Source: three-view drawing plus pictorial views. Frame: mm from the lowest corner of the part. A direction names the side the tool comes from. Round coordinates to 2 decimals unless told otherwise and drop trailing zeros. Order: outer loops, then holes, each group sorted by start corner. A loop starts at its lowest first (then second) coordinate and runs counter-clockwise, first axis right, second up. Notation, with made-up numbers: M 38,79 L 42,79 A18 cw 42,90 Z; hole C 48,10 d6. An arc over 180 degrees is marked long. Return JSON: item names as keys, results as strings. Group by question number.
Q1. Mould query, pull axis Y, two halves, no side actions, for the marked faces 1, 2 and 3. Classes: released by +Y, released by -Y, zero draft, split by the parting line, or undercut.
Q2. Ray query, probe 1 along Y at (x, z) = (12, 4.25); probe 2 along X at (y, z) = (11, 1.5); probe 3 along Y at (x, z) = (70, 0.75). Return the intervals inside material, ascending.
Q3. Access query for the marked faces 4 and 5. Directions: +Z, -Z, +X, -X, +Y, -Y. A direction counts if a zero-diameter tool reaches every point of the face in a straight line with its end or side. Return the directions, or none.
Q4. Cut plane D-D on x = 23.5. Output: boundary loops of the cut face in (y, z), and give its area (3 significant figures).
Q5. Contact query for flat-ended pins moving along their axis: pin 1 (1 mm diameter, centred on x = 31, y = 17.5, fed in from +Z); pin 2 (3.5 mm diameter, centred on x = 45, y = 12.5, fed in from +Z). Output: stop coordinate, or through.
Q6. Cut plane B-B on z = 20. Output: boundary loops of the cut face in (x, y).
Q7. Cut plane C-C on x = 35. Output: boundary loops of the cut face in (y, z).
Q8. Cut plane A-A on y = 12.5. Output: boundary loops of the cut face in (x, z), and give its area (3 significant figures).
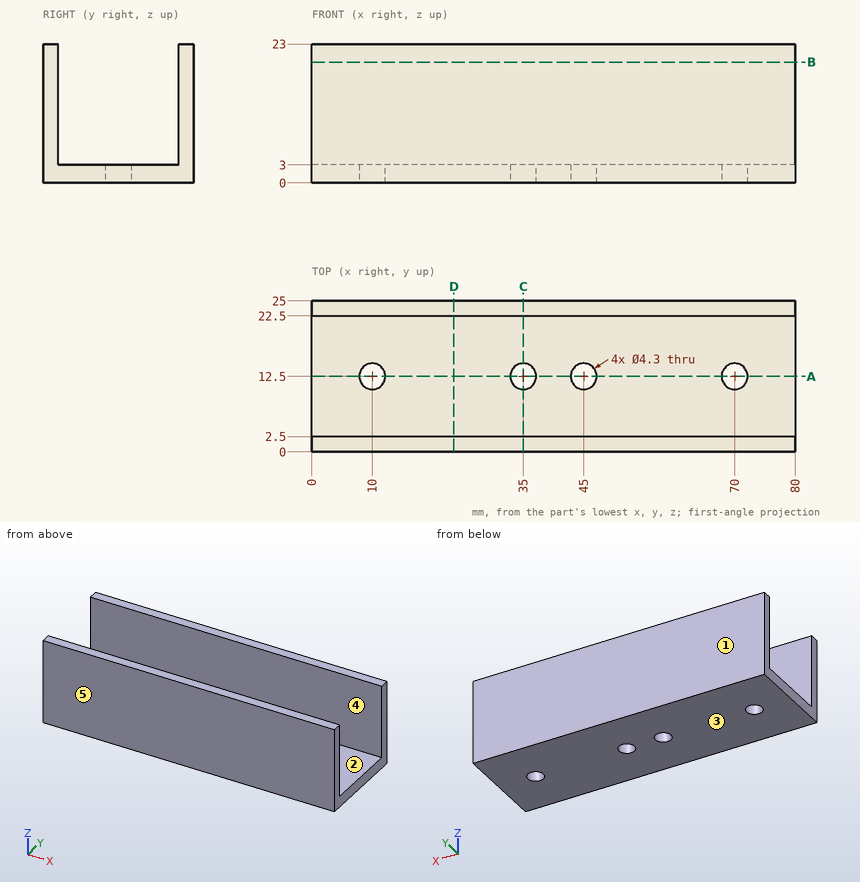
Result sheet:
{
 "1": {"face 1": "released by +Y", "face 2": "undercut", "face 3": "zero draft"},
 "2": {"probe 1": "y = 0 to 2.5, 22.5 to 25", "probe 2": "x = 0 to 8.46, 11.54 to 33.46, 36.54 to 43.46, 46.54 to 68.46, 71.54 to 80", "probe 3": "y = 0 to 10.35, 14.65 to 25"},
 "3": {"face 4": "+Z, +X, -X", "face 5": "+Z, -Z, +X, -X, -Y"},
 "4": {"outline": "M 0,0 L 25,0 L 25,23 L 22.5,23 L 22.5,3 L 2.5,3 L 2.5,23 L 0,23 Z", "area": "175 mm²"},
 "5": {"pin 1": "stops at z = 3", "pin 2": "passes through"},
 "6": {"outline": "M 0,0 L 80,0 L 80,2.5 L 0,2.5 Z; M 0,22.5 L 80,22.5 L 80,25 L 0,25 Z"},
 "7": {"outline": "M 0,0 L 10.35,0 L 10.35,3 L 2.5,3 L 2.5,23 L 0,23 Z; M 14.65,0 L 25,0 L 25,23 L 22.5,23 L 22.5,3 L 14.65,3 Z"},
 "8": {"outline": "M 0,0 L 7.85,0 L 7.85,3 L 0,3 Z; M 12.15,0 L 32.85,0 L 32.85,3 L 12.15,3 Z; M 37.15,0 L 42.85,0 L 42.85,3 L 37.15,3 Z; M 47.15,0 L 67.85,0 L 67.85,3 L 47.15,3 Z; M 72.15,0 L 80,0 L 80,3 L 72.15,3 Z", "area": "188 mm²"}
}
